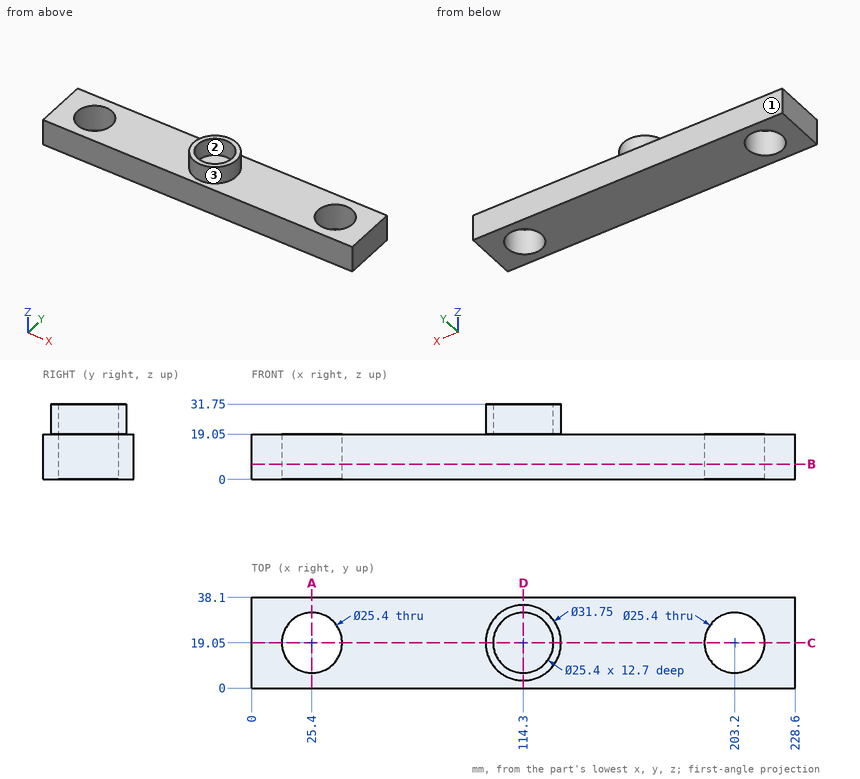
Input: dimensioned drawing with shaded views. Units: mm. Origin: part minimum x, y, z. Round coordinates to 2 decimals unless told otherwise and drop trailing zeros. Loops run counter-clockwise (first coordinate to the right, second up) from the corner with the lowest first, then second, coordinate; pieces in that order, holes last. Notation, with made-up numbers: M 17,78 L 24,78 A15 ccw 24,96 Z; hole C 48,-34.5 d9. An arc over 180 degrees is marked long. Return JSON: item names as keys, results as strings. Group by question number.
1. Material intervals for line 1 along X through (y, z) = (19, 4); line 2 along Y through (x, z) = (114, 24); line 3 along X through (y, z) = (27, 9), sorted ascending. Write a range as from..to.
2. Section query A-A on x = 25.4. Output: boundary loops of the cut face in (y, z), and give its area (3 significant figures).
3. Section query C-C on y = 19.05. Output: boundary loops of the cut face in (x, z) (3 decimals), and give its area (3 significant figures).
4. Mould query, pull axis Y, two halves, no side actions, for the marked faces 1, 2 and 3. Classes: released by +Y, released by -Y, zero draft, split by the parting line, or undercut.
5. Pin query (flat end, axial travel): pin 1 (11.5 mm diameter, centred on x = 154, y = 20, fed in from +Z); pin 2 (20.5 mm diameter, centred on x = 203.2, y = 19.05, fed in from +Z). Return the tip coordinate at first contact, or that it passes through.
6. Section query D-D on x = 114.3. Output: boundary loops of the cut face in (y, z) (3 decimals), and give its area (3 significant figures).
7. Section query B-B on z = 6.5. Output: boundary loops of the cut face in (x, y), and give its area (3 significant figures).
Checks:
{
 "1": {"line 1": "x = 0..12.7, 38.1..190.5, 215.9..228.6", "line 2": "y = 3.18..6.35, 31.75..34.92", "line 3": "x = 0..15.5, 35.3..193.3, 213.1..228.6"},
 "2": {"outline": "M 0,0 L 6.35,0 L 6.35,19.05 L 0,19.05 Z; M 31.75,0 L 38.1,0 L 38.1,19.05 L 31.75,19.05 Z", "area": "242 mm²"},
 "3": {"outline": "M 0,0 L 12.7,0 L 12.7,19.05 L 0,19.05 Z; M 38.1,0 L 190.5,0 L 190.5,19.05 L 130.175,19.05 L 130.175,31.75 L 127,31.75 L 127,19.05 L 101.6,19.05 L 101.6,31.75 L 98.425,31.75 L 98.425,19.05 L 38.1,19.05 Z; M 215.9,0 L 228.6,0 L 228.6,19.05 L 215.9,19.05 Z", "area": "3,470 mm²"},
 "4": {"face 1": "released by +Y", "face 2": "undercut", "face 3": "split by the parting line"},
 "5": {"pin 1": "stops at z = 19.05", "pin 2": "passes through"},
 "6": {"outline": "M 0,0 L 38.1,0 L 38.1,19.05 L 34.925,19.05 L 34.925,31.75 L 31.75,31.75 L 31.75,19.05 L 6.35,19.05 L 6.35,31.75 L 3.175,31.75 L 3.175,19.05 L 0,19.05 Z", "area": "806 mm²"},
 "7": {"outline": "M 0,0 L 228.6,0 L 228.6,38.1 L 0,38.1 Z; hole C 25.4,19.05 d25.4; hole C 203.2,19.05 d25.4", "area": "7,700 mm²"}
}
